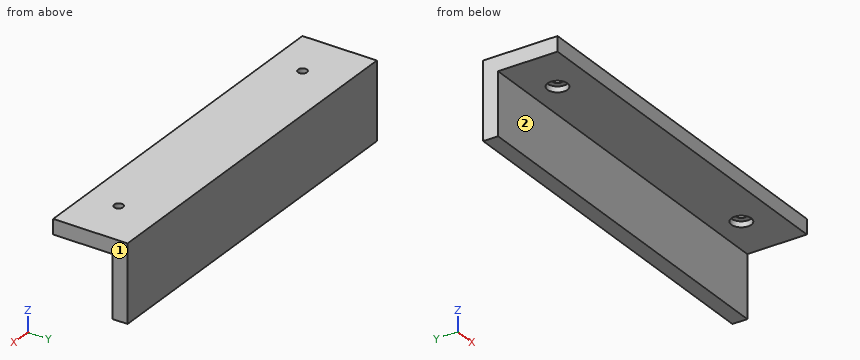
from build123d import *

# Parameters (mm, degrees)
F0_W     = 150
F0_H     = 25
F0_H_2   = 6
F1_DEPTH = 6
F2_DEPTH = 30
F3_R     = 4
F3_R_2   = 1.8
F4_DEPTH = 27.31
F5_DEPTH = 25


with BuildPart() as f1:
    # F0 (on Front) → F1 (new body)
    with BuildSketch(Plane.XZ):
        with Locations((36.419376108, 12.5)):
            Rectangle(F0_W, F0_H)
        with Locations((36.419376108, 28)):
            Rectangle(F0_W, F0_H_2)
    extrude(amount=F1_DEPTH)

    # F0 (on Front) → F2 (join)
    with BuildSketch(Plane.XZ):
        with Locations((36.419376108, 28)):
            Rectangle(F0_W, F0_H_2)
    extrude(amount=F2_DEPTH)

    # F3 (on Top) → F4 (cut)
    with BuildSketch(Plane.XY):
        with Locations((91.85885638, -16.7120620608)):
            Circle(F3_R)
        with Locations((91.8588588197, -16.7120620608)):
            Circle(F3_R_2, mode=Mode.SUBTRACT)
        with Locations((-18.8037762601, -16.7120620608)):
            Circle(F3_R)
        with Locations((-18.8037762601, -16.7120620608)):
            Circle(F3_R_2, mode=Mode.SUBTRACT)
    extrude(amount=F4_DEPTH, mode=Mode.SUBTRACT)

    # F5 (cut): faces of the model
    f5_faces = [f1.faces().sort_by_distance(p)[0] for p in [
        (-18.8037762601, -16.7120620608, 25),
        (91.8588588197, -16.7120620608, 25),
    ]]
    extrude(f5_faces, amount=-F5_DEPTH, mode=Mode.SUBTRACT)


solid = f1.part
Verification items for the finished model (mm, model axes). Face numbers are marked on the shaded views. A direction names the side the tool comes from. Give positions to 0.01 mm unless a question says otherwise; leave off trailing zeros. Order: outer loops, then holes, each group sorted by start corner. A loop starts at its lowest first (then second) coordinate and runs counter-clockwise, first axis right, second up. Notation, with made-up numbers: M 38,-1.75 L 80,-1.75 A23 ccw 80,30.25 Z; hole C -22,-8.5 d2. An arc over 180 degrees is marked long. Answer as a JSON object with one key per item and string values. Group by question number.
1) Access from +Z, -Z, +X, -X, +Y, -Y to the whole of each face (thin tool, end or side, straight path). Record for the marked faces 1 and 2.
2) Cross-section at A-A (x = 92). Enter the section's corners in (y, z), then the cut area to 3 significant figures.
3) Cross-section at D-D (y = -8). Enter the section's corners in (x, z), then the cut area to 3 significant figures.
4) Cross-section at C-C (x = 64). Enter the section's corners in (y, z), then the cut area to 3 significant figures.
5) Cross-section at B-B (z = 20). Enter the section's corners in (x, y), then the cut area to 3 significant figures.
6) Depth check by flat-ended pin: pin 1 Ø12 at (x, z) = (32, 4.5) entering from -Y; pin 2 Ø9 at (x, y) = (92, -15) entering from -Z; pin 3 Ø4.5 at (x, y) = (-18.8, -16.71) entering from -Z. Enter the tip coordinate at first touch or a pass-through.
7) Scan lines: line 1 along X through (y, z) = (-17, 29.5); line 2 along X through (y, z) = (-18.75, 27); line 3 along Y through (x, z) = (3, 5). Record each from-to range of solid material in increasing order. Write a range as [from, to].
Result sheet:
{
 "1": {"face 1": "+Z, -Z, +X, +Y, -Y", "face 2": "-Z, +X, -X, -Y"},
 "2": {"outline": "M -30,25 L -20.71,25 L -20.71,27.31 L -18.51,27.31 L -18.51,31 L -30,31 Z; M -14.92,27.31 L -12.71,27.31 L -12.71,25 L -6,25 L -6,0 L 0,0 L 0,31 L -14.92,31 Z", "area": "298 mm2"},
 "3": {"outline": "M -38.58,25 L 111.42,25 L 111.42,31 L -38.58,31 Z", "area": "900 mm2"},
 "4": {"outline": "M -30,25 L -6,25 L -6,0 L 0,0 L 0,31 L -30,31 Z", "area": "330 mm2"},
 "5": {"outline": "M -38.58,-6 L 111.42,-6 L 111.42,0 L -38.58,0 Z", "area": "900 mm2"},
 "6": {"pin 1": "stops at y = -6", "pin 2": "stops at z = 25", "pin 3": "stops at z = 27.31"},
 "7": {"line 1": "x = [-38.58, -20.58], [-17.03, 90.08], [93.64, 111.42]", "line 2": "x = [-38.58, -22.25], [-15.36, 88.42], [95.3, 111.42]", "line 3": "y = [-6, 0]"}
}
